Could you check a few things on this model? Use its own coordinates, in mm. Face numbers are marked on the shaded views. A direction names the side the tool comes from. Coordinates: 2 decimals unless noted, no trailing zeros. Write each loop counter-clockwise with the first axis right and the second up, starting at its lowest first coordinate (ties: lowest second). Pieces come first, ordered by that corner, then holes. Notation, with made-up numbers: M 9,10 L 44,10 A25 cw 44,35 Z; hole C 25.5,-19.75 d9. An arc over 180 degrees is marked long. Write item = value, one per line.
Autodesk Inventor part; units mm, degrees
ref_plane "YZ Plane" through (0, 0, 0) normal (1, 0, 0) x (0, 1, 0)
ref_plane "XZ Plane" through (0, 0, 0) normal (0, 1, 0) x (-1, 0, 0)
ref_plane "XY Plane" through (0, 0, 0) normal (0, 0, 1) x (1, 0, 0)
sketch "Náčrt1" plane through (0, 0, 0) normal (0, 1, 0) x (-1, 0, 0)
  line L0 (2.45, 6.925) -> (-2.45, 6.925)
  line L1 (-2.45, 6.925) -> (-2.45, 3.025)
  line L2 (-2.45, 3.025) -> (2.45, 3.025)
  line L3 (2.45, 3.025) -> (2.45, 6.925)
  line L4 (2.45, -3.025) -> (-2.45, -3.025)
  line L5 (-2.45, -3.025) -> (-2.45, -6.925)
  line L6 (-2.45, -6.925) -> (2.45, -6.925)
  line L7 (2.45, -6.925) -> (2.45, -3.025)
  point P0 (0, 0)
  dimension "d0" = 6.05
  dimension "d1" = 3.9
  dimension "d2" = 3.9
  dimension "d3" = 4.9
  dimension "d4" = 4.9
  dimension "d5" = 2.45
  dimension "d6" = 3.025
extrude "Vysunutí1" add sketch "Náčrt1" along normal blind 7
sketch "Náčrt2" plane through (0, 7, 0) normal (0, 1, 0) x (1, 0, 0)
  line L0 (-3.95, -8.425) -> (3.95, -8.425)
  line L1 (3.95, -8.425) -> (3.95, 8.425)
  line L2 (3.95, 8.425) -> (-3.95, 8.425)
  line L3 (-3.95, 8.425) -> (-3.95, -8.425)
  line L4 (-2.45, -3.025) -> (-2.45, -6.925)
  line L5 (-2.45, -6.925) -> (2.45, -6.925)
  line L6 (2.45, 6.925) -> (-2.45, 6.925)
  line L7 (2.45, 3.025) -> (2.45, 6.925)
  point P0 (0, 0)
  dimension "d9" = 1.5
  dimension "d10" = 1.5
  dimension "d11" = 1.5
  dimension "d12" = 1.5
extrude "Vysunutí2" add sketch "Náčrt2" along normal blind 11
sketch "Náčrt3" plane through (0, 18, 0) normal (0, 1, 0) x (1, 0, 0)
  line L0 (-3.95, -8.425) -> (3.95, -8.425)
  line L1 (3.95, -8.425) -> (3.95, 8.425)
  line L2 (-3.95, 8.425) -> (-3.95, -8.425)
  line L3 (-7, 0) -> (18, 25)
  line L4 (18, 25) -> (43, 0)
  line L5 (43, 0) -> (18, -25)
  line L6 (18, -25) -> (-7, 0)
  line L7 (3.95, 8.425) -> (-3.95, 8.425)
  line L8 (3.95, 8.425) -> (-3.95, 8.425)
  point P0 (0, 0)
  point P1 (3.95, -8.0855)
  point P2 (3.95, 8.1088)
  point P3 (1.425, -8.425)
  point P4 (1.425, 8.425)
  point P5 (-3.95, 3.05)
  point P6 (-3.95, -3.05)
  dimension "d22" = 90
  dimension "d24" = 90
  dimension "d25" = 135
  dimension "d30" = 7
  dimension "d32" = 0
  dimension "d33" = 25
  dimension "d34" = 25
  dimension "d35" = 3.95
  dimension "d36" = 3.05
  dimension "d40" = 90
extrude "Vysunutí4" add sketch "Náčrt3" along normal blind 1
fillet "Zaoblení1" radius 1.2 4 edges at (-3.95, 13, 8.425) (3.95, 12.5, 8.425) (3.95, 12.5, -8.425) (-3.95, 13, -8.425)
equation "\"d2\" = d1"
equation "\"d4\" = d3"
equation "\"d10\" = d9"
equation "\"d11\" = d9"
equation "\"d12\" = d10"
equation "\"d24\" = d22"
properties part number "QRholder-top"
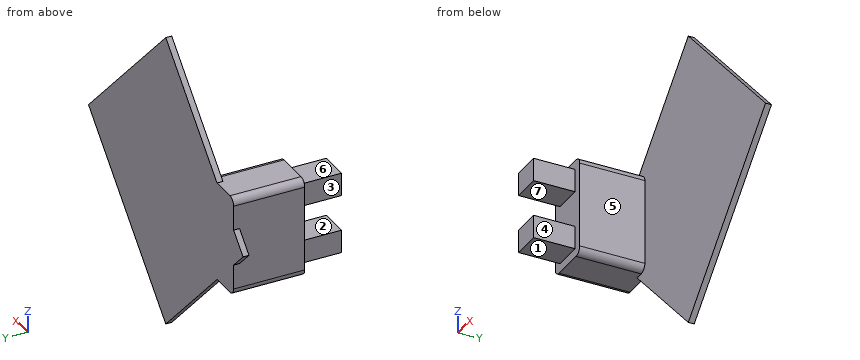
Item 1: I'm going to push flat-ended pins straight in: P1, Ø1.2, axis at y = 5, z = -5, coming from the +X side; P2, Ø1.5, axis at x = 1, y = 4, coming from the -Z side (3 decimals); P3, Ø1.2, axis at y = 4, z = -5, coming from the -X side; P4, Ø10, axis at y = 12, z = 19.5, coming from the -X side. Where does each tip first touch, or does it pass through?
Numbers:
P1 = 2.45
P2 = -6.925
P3 = -2.45
P4 = through
Item 2: If we mould it in two halves opening along Z, with no side actions, what happens to the marked faces 5, 6 and 7? For each: pulls with the +Z half, pulls with the -Z half, needs draft (parallel to the pull), parting line crosses it, or undercut.
Numbers:
face_5 = needs draft
face_6 = pulls with the +Z half
face_7 = undercut
Item 3: Imagine slicing it at B-B (y = 2). Write out the boundary of the cut face in (x, z) (3 decimals), and give its area (3 significant figures).
Numbers:
outline = M -2.45,-6.925 L 2.45,-6.925 L 2.45,-3.025 L -2.45,-3.025 Z; M -2.45,3.025 L 2.45,3.025 L 2.45,6.925 L -2.45,6.925 Z
area = 38.2 mm²
Item 4: Imagine slicing it at C-C (x = -0.5). Write out the boundary of the cut face in (y, z) (3 decimals), and give its area (3 significant figures).
Numbers:
outline = M 0,-6.925 L 7,-6.925 L 7,-8.425 L 19,-8.425 L 19,8.425 L 7,8.425 L 7,6.925 L 0,6.925 L 0,3.025 L 7,3.025 L 7,-3.025 L 0,-3.025 Z
area = 257 mm²
Item 5: Imagine slicing it at D-D (y = 13.5). Write out the boundary of the cut face in (x, z) (3 decimals), and give its area (3 significant figures).
Numbers:
outline = M -3.95,-7.225 A1.2 ccw -2.75,-8.425 L 2.75,-8.425 A1.2 ccw 3.95,-7.225 L 3.95,7.225 A1.2 ccw 2.75,8.425 L -2.75,8.425 A1.2 ccw -3.95,7.225 Z
area = 132 mm²
Item 6: Imagine slicing it at A-A (z = -5.5). Write out the boundary of the cut face in (x, y), and give its area (3 significant figures).
Numbers:
outline = M -3.95,7 L -2.45,7 L -2.45,0 L 2.45,0 L 2.45,7 L 3.95,7 L 3.95,18 L 37.5,18 L 37.5,19 L -3.95,19 Z
area = 163 mm²
Item 7: If I drill on line 1 along X through (y, z) = (1.25, -5); line 2 along Y through (x, z) = (3, -9.5); line 3 along X through (y, z) = (10, -7), over which ranges is the centre line in solid material (lowest first)?
Numbers:
line_1 = -2.45 to 2.45
line_2 = 18 to 19
line_3 = -3.95 to 3.95
Item 8: For the marked faces 1, 2, 3 and 4, which set-ups out of +Z, -Z, +X, -X, +Y, -Y let a thin tool reach every point of the face, with its end or its side?
Numbers:
face_1 = -Z, +X, -X, -Y
face_2 = +X, -X, -Y
face_3 = +Z, -Z, -X, -Y
face_4 = +Z, -Z, +X, -Y
